Autodesk Inventor part; units mm, degrees
ref_plane "Počáteční rovina" through (0, 0, 0) normal (0, 0, 1) x (1, 0, 0)
ref_plane "Koncová rovina" through (0, 0, 250) normal (0, 0, 1) x (1, 0, 0)
ref_plane "YZ Plane" through (0, 0, 0) normal (1, 0, 0) x (0, 1, 0)
ref_plane "Počáteční rovina" through (0, 0, 0) normal (0, 0, 1) x (1, 0, 0)
ref_plane "Koncová rovina" through (0, 0, 250) normal (0, 0, 1) x (1, 0, 0)
sketch "Náčrt1" plane through (0, 0, 0) normal (0, 0, 1) x (1, 0, 0)
  line L0 (-11.5, 17.5) -> (11.5, 17.5)
  line L1 (17.5, 11.5) -> (17.5, -11.5)
  line L2 (11.5, -17.5) -> (-11.5, -17.5)
  line L3 (-17.5, -11.5) -> (-17.5, 11.5)
  arc A0 (-11.5, 17.5) -> (-17.5, 11.5) centre (-11.5, 11.5) ccw
  arc A1 (17.5, 11.5) -> (11.5, 17.5) centre (11.5, 11.5) ccw
  arc A2 (11.5, -17.5) -> (17.5, -11.5) centre (11.5, -11.5) ccw
  arc A3 (-17.5, -11.5) -> (-11.5, -17.5) centre (-11.5, -11.5) ccw
  line L4 (-26.2397, 0) -> (26.2397, 0) construction
  line L5 (0, -26.2397) -> (0, 26.2397) construction
  arc A4 (-11.5, 14.5) -> (-14.5, 11.5) centre (-11.5, 11.5) ccw
  line L6 (-11.5, 14.5) -> (11.5, 14.5)
  arc A5 (14.5, 11.5) -> (11.5, 14.5) centre (11.5, 11.5) ccw
  line L7 (14.5, 11.5) -> (14.5, -11.5)
  arc A6 (11.5, -14.5) -> (14.5, -11.5) centre (11.5, -11.5) ccw
  line L8 (11.5, -14.5) -> (-11.5, -14.5)
  arc A7 (-14.5, -11.5) -> (-11.5, -14.5) centre (-11.5, -11.5) ccw
  line L9 (-14.5, -11.5) -> (-14.5, 11.5)
  point P0 (-17.5, 17.5)
  point P1 (17.5, -17.5)
  point P2 (17.5, 17.5)
  dimension "b" = 35
  dimension "msp_r" = 6
  dimension "d8" = 17.5
  dimension "d9" = 17.5
  dimension "d10" = 3
extrude "Těleso" add sketch "Náčrt1" along normal blind 247.5
sketch "Sketch2" plane through (0, 0, 0) normal (0, 0, 1) x (1, 0, 0)
  line L0 (0, 0) -> (10, 0)
ref_plane "Work Plane3" through (0, 0, 0) normal (0, -1, 0) x (1, 0, 0)
sketch "Sketch3" plane through (0, 0, 0) normal (0, -1, 0) x (1, 0, 0)
  line L0 (-2, 0) -> (12, 0)
  line L1 (-2, 250) -> (12, 250)
  dimension "d14" = 250
equation "\"msp_r\" = 2 * ParT"
equation "\"d8\" = d9"
equation "\"d9\" = 0.5 * b"
equation "\"d10\" = ParT"
equation "\"G_OFFSET_START\" = 0"
equation "\"G_OFFSET_END\" = 0"
equation "\"G_L\" = d14"
properties part number "CSN 426935 - 35x35x3-250" material "Nerezová ocel"
CAD build for the part. Positions are in the model's coordinates, mm. A direction names the side the tool comes from. Round coordinates to 2 decimals unless told otherwise and drop trailing zeros. Write each loop counter-clockwise with the first axis right and the second up, starting at its lowest first coordinate (ties: lowest second). Pieces come first, ordered by that corner, then holes.
(1) 3-axis set-ups, long thin cutter, end or side, ignore diameter. For faces 4 (the face through (0, 17.5, 122)), 5 (the face through (0, -14.5, 122)): which of +Z, -Z, +X, -X, +Y, -Y reach the whole face in a straight line?
(2) Slice it at A-A, the plane x = 3. Write the cut outline in (y, z).
(3) Slice it at C-C, the plane z = 175.5. Write the cut outline in (x, y).
(4) Probe line 1 along X through (y, z) = (-7, 104); line 2 along Y through (x, z) = (-13.5, 138.5). List the from-to ranges inside material, lowest first.
(5) Drop flat-ended pins along their axis: P1, Ø4, axis at x = 12, y = 12, coming from the +Z side; P2, Ø3, axis at y = -14, z = 62, coming from the +X side. Give the stop position or say it passes through.
(6) Mould opens along X. For faces 1 (the face through (-15.789, 15.696, 122.018)), 2 (the face through (-14.5, 0, 122)), 3 (the face through (15.696, 15.789, 122.018)) say: pulls with the +X half, pulls with the -X half, needs draft (parallel to the pull), parting line crosses it, or undercut.
From the geometry:
1. face 4: +Z, -Z, +X, -X, +Y
1. face 5: +Z, -Z
2. outline: (-17.5, 0) - (-14.5, 0) - (-14.5, 247.5) - (-17.5, 247.5) - close; (14.5, 0) - (17.5, 0) - (17.5, 247.5) - (14.5, 247.5) - close
3. outline: (-17.5, -11.5) arc R6 ccw to (-11.5, -17.5) - (11.5, -17.5) arc R6 ccw to (17.5, -11.5) - (17.5, 11.5) arc R6 ccw to (11.5, 17.5) - (-11.5, 17.5) arc R6 ccw to (-17.5, 11.5) - close; hole (-14.5, -11.5) arc R3 ccw to (-11.5, -14.5) - (11.5, -14.5) arc R3 ccw to (14.5, -11.5) - (14.5, 11.5) arc R3 ccw to (11.5, 14.5) - (-11.5, 14.5) arc R3 ccw to (-14.5, 11.5) - close
4. line 1: x = -17.5 to -14.5, 14.5 to 17.5
4. line 2: y = -17.16 to -13.74, 13.74 to 17.16
5. P1: passes through
5. P2: stops at x = 17.42
6. face 1: pulls with the -X half
6. face 2: undercut
6. face 3: pulls with the +X half
